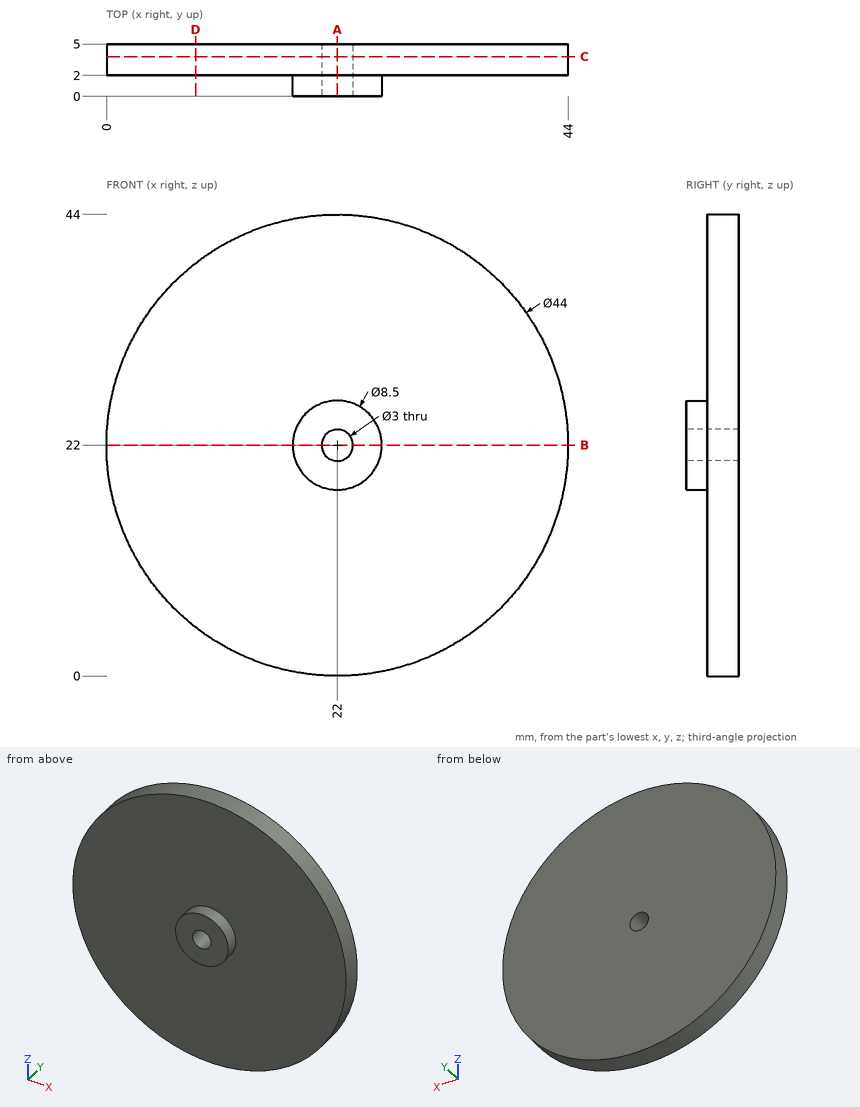
Source: three-view drawing plus pictorial views. Frame: mm from the lowest corner of the part. Give positions to 0.01 mm unless a question says otherwise; leave off trailing zeros. Write each loop counter-clockwise with the first axis right and the second up, starting at its lowest first coordinate (ties: lowest second). Pieces come first, ordered by that corner, then holes.
(1) Cut plane D-D, the plane x = 8.5. Return loops of the section in (y, z).
(2) First-contact query: P1, Ø3, axis at x = 22, y = 4, coming from the +Z side; P2, Ø1.5, axis at y = 4, z = 19.5, coming from the +X side. Flat tips, straight axial feed; report the tip coordinate or a pass-through.
(3) Ray query, line 1 (Z direction, x = 22, y = 2.5); line 2 (Y direction, x = 29, z = 16); line 3 (X direction, y = 2.9, z = 30). Return the intervals inside material, ascending.
(4) Cut plane A-A, the plane x = 22. Return loops of the section in (y, z).
(5) Cut plane C-C, the plane y = 3.8. Return loops of the section in (x, z), then the cut area to 3 significant figures.
(6) Cut plane B-B, the plane z = 22. Return loops of the section in (x, y).
Values follow:
1. outline: (2, 4.63) - (5, 4.63) - (5, 39.37) - (2, 39.37) - close
2. P1: stops at z = 44
2. P2: stops at x = 43.93
3. line 1: z = 0 to 20.5, 23.5 to 44
3. line 2: y = 2 to 5
3. line 3: x = 1.51 to 42.49
4. outline: (0, 17.75) - (2, 17.75) - (2, 0) - (5, 0) - (5, 20.5) - (0, 20.5) - close; (0, 23.5) - (5, 23.5) - (5, 44) - (2, 44) - (2, 26.25) - (0, 26.25) - close
5. outline: circle Ø44 at (22, 22); hole circle Ø3 at (22, 22)
5. area: 1,510 mm2
6. outline: (0, 2) - (17.75, 2) - (17.75, 0) - (20.5, 0) - (20.5, 5) - (0, 5) - close; (23.5, 0) - (26.25, 0) - (26.25, 2) - (44, 2) - (44, 5) - (23.5, 5) - close
